from build123d import *

# Parameters (mm, degrees)
SKETCH1_R           = 4
BOSS_EXTRUDE2_DEPTH = 0.5
FILLET1_R           = 10
SKETCH3_R           = 1
CUT_EXTRUDE2_DEPTH  = 1.5


with BuildPart() as part:
    # Sketch1 → Boss-Extrude2 (new body)
    with BuildSketch(Plane(origin=(0, 0, 0), x_dir=(1, 0, 0), z_dir=(0, 1, 0))):
        with BuildLine():
            Line((7.464101615, 2), (3.464101615, 2))
            ThreePointArc((3.464101615, 2), (3.863703305, 1.03527618), (4, 0))
            ThreePointArc((4, 0), (3.863703305, -1.03527618), (3.464101615, -2))
            Line((3.464101615, -2), (7.464101615, -2))
            Line((7.464101615, -2), (11.302617333, -4.027174803))
            Line((11.302617333, -4.027174803), (31.492947109, 0))
            Line((31.492947109, 0), (11.302617333, 4.027174803))
            Line((11.302617333, 4.027174803), (7.464101615, 2))
        make_face()
        Circle(SKETCH1_R)
    extrude(amount=BOSS_EXTRUDE2_DEPTH)

    # Fillet1
    fillet1_edges = [part.edges().sort_by_distance(p)[0] for p in [
        (3.464101615, 0.25, 2),
        (3.464101615, 0.25, -2),
    ]]
    fillet(fillet1_edges, radius=FILLET1_R)

    # Sketch3 → Cut-Extrude2 (cut, through all)
    with BuildSketch(Plane(origin=(0, 0.5, 0), x_dir=(1, 0, 0), z_dir=(0, 1, 0))):
        Circle(SKETCH3_R)
    extrude(amount=-CUT_EXTRUDE2_DEPTH, mode=Mode.SUBTRACT)


solid = part.part
Check sheet for the modelled part. Datum: model origin and axes. Units: mm. A direction names the side the tool comes from. Round coordinates to 2 decimals unless told otherwise and drop trailing zeros. Loops run counter-clockwise (first coordinate to the right, second up) from the corner with the lowest first, then second, coordinate; pieces in that order, holes last. Notation, with made-up numbers: (80.25, 76.25) - (121.25, 76.25) arc R24 ccw to (121.25, 115.25) - close; hole circle Ø8 at (59.25, -2.75). An arc over 180 degrees is marked (long way). Answer as CSV lines item,"result". Start each with the question number.
Item 1: Section check C-C (z = 3). Record the boundary of the cut face in (x, y), and give its area (3 significant figures).
Item 2: Section check D-D (x = 18). Record the boundary of the cut face in (y, z), and give its area (3 significant figures).
Item 3: Scan lines: line 1 (Z direction, x = 0, y = 0.35); line 2 (Z direction, x = 4.5, y = 0.2); line 3 (Z direction, x = 27.5, y = 0.25). Record each from-to range of solid material in increasing order. Write a range as [from, to].
Item 4: Section check B-B (x = 0). Record the boundary of the cut face in (y, z), and give its area (3 significant figures).
Item 5: Section check A-A (y = 0.4). Record the boundary of the cut face in (x, z).
Item 6: Set-up check for faces 4 (the flat face through (9.36, 0.25, 3)), 5 (the flat face through (21.26, 0.25, 2.04)), 6 (the flat face through (9.41, 0.246, -3.028)): record each of +Z, -Z, +X, -X, +Y, -Y from which the full face is reachable in a straight line by a thin tool's end or side.
Item 7: Release check for a two-part mould opening along Z. For faces 1 (the flat face through (10, 0, 0)), 2 (the cylindrical face through (-0.217, 0.254, 0.976)), 3 (the cylindrical face through (4.502, 0.254, 2.374)) record: +Z half, -Z half, draft (parallel to the pull), parting line (faces both ways), or undercut.
Report:
1,outline,"(-2.65, 0) - (2.85, 0) - (2.85, 0.5) - (-2.65, 0.5) - close; (9.36, 0) - (16.45, 0) - (16.45, 0.5) - (9.36, 0.5) - close"
1,area,"6.30 mm2"
2,outline,"(0, -2.69) - (0.5, -2.69) - (0.5, 2.69) - (0, 2.69) - close"
2,area,"2.69 mm2"
3,line 1,"z = [-4, -1], [1, 4]"
3,line 2,"z = [-2.37, 2.37]"
3,line 3,"z = [-0.8, 0.8]"
4,outline,"(0, -4) - (0.5, -4) - (0.5, -1) - (0, -1) - close; (0, 1) - (0.5, 1) - (0.5, 4) - (0, 4) - close"
4,area,"3.00 mm2"
5,outline,"(2.06, -3.43) arc R10 cw to (7.21, -2) - (7.46, -2) - (11.3, -4.03) - (31.49, 0) - (11.3, 4.03) - (7.46, 2) - (7.21, 2) arc R10 cw to (2.06, 3.43) arc R4 ccw (long way) to start; hole circle Ø2 at (0, 0)"
6,face 4,"+Z, +Y, -Y"
6,face 5,"+Z, +X, +Y, -Y"
6,face 6,"-Z, +Y, -Y"
7,face 1,"draft"
7,face 2,"undercut"
7,face 3,"+Z half"
